For this review, use the dimensioned drawing (mm, ordinates from the lowest corner) and the shaded views. A direction names the side the tool comes from. Coordinates: 2 decimals unless noted, no trailing zeros. Loops run counter-clockwise (first coordinate to the right, second up) from the corner with the lowest first, then second, coordinate; pieces in that order, holes last. Notation, with made-up numbers: M 37,22 L 69,22 A24 ccw 69,38 Z; hole C -25,47 d10. An arc over 180 degrees is marked long. Write item = value, one per line.
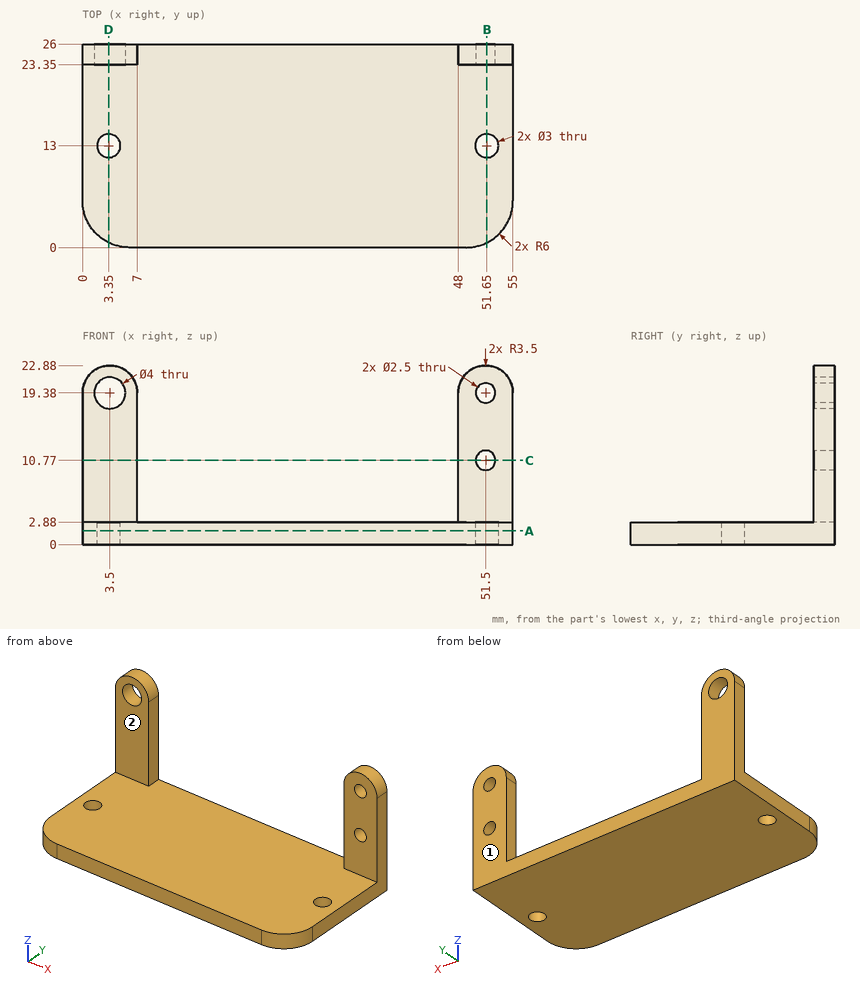
Q1. Machinability: for the marked faces 1 and 2, which of the approach directions +Z, -Z, +X, -X, +Y, -Y give a long, thin tool a straight path to every point of the face, cutting with its end or side? Answer none if there is none.
Solved:
face_1 = +Z, -Z, +X, -X, +Y
face_2 = +Z, +X, -X, -Y
Q2. Add section A-A (z = 1.75). Write out the cut boundary in (x, y), and give its area (3 significant figures).
Solved:
outline = M 0,6 A6 ccw 6,0 L 49,0 A6 ccw 55,6 L 55,26 L 0,26 Z; hole C 3.35,13 d3; hole C 51.65,13 d3
area = 1,400 mm²
Q3. For line 1 along Z through (x, y) = (51.5, 24.85); line 2 along Z through (x, y) = (45, 16); line 3 along Z through (x, y) = (3.5, 24.65), list the stretches that pass through material, from the lowest coordinate up.
Solved:
line_1 = 0 to 9.52, 12.02 to 18.13, 20.63 to 22.88
line_2 = 0 to 2.88
line_3 = 0 to 17.38, 21.38 to 22.88
Q4. For pin 1 Ø5 at (x, y) = (16, 12.5) entering from +Z; pin 2 Ø2 at (x, z) = (51.5, 16) entering from -Y; pin 3 Ø10 at (y, z) = (16, 15) entering from +X, all flat-tipped, find the tip position at first contact; note any pin that passes through.
Solved:
pin_1 = 2.88
pin_2 = 23.35
pin_3 = through
Q5. Add section C-C (z = 10.77). Write out the cut boundary in (x, y), and give its area (3 significant figures).
Solved:
outline = M 0,23.35 L 7,23.35 L 7,26 L 0,26 Z; M 48,23.35 L 50.25,23.35 L 50.25,26 L 48,26 Z; M 52.75,23.35 L 55,23.35 L 55,26 L 52.75,26 Z
area = 30.5 mm²
Q6. Add section D-D (x = 3.35). Write out the cut boundary in (y, z), and give its area (3 significant figures).
Solved:
outline = M 0.62,0 L 11.5,0 L 11.5,2.88 L 0.62,2.88 Z; M 14.5,0 L 26,0 L 26,17.39 L 23.35,17.39 L 23.35,2.88 L 14.5,2.88 Z; M 23.35,21.37 L 26,21.37 L 26,22.88 L 23.35,22.88 Z
area = 107 mm²
Q7. Add section B-B (x = 51.65). Write out the cut boundary in (y, z).
Solved:
outline = M 0.62,0 L 11.5,0 L 11.5,2.88 L 0.62,2.88 Z; M 14.5,0 L 26,0 L 26,9.53 L 23.35,9.53 L 23.35,2.88 L 14.5,2.88 Z; M 23.35,12.01 L 26,12.01 L 26,18.14 L 23.35,18.14 Z; M 23.35,20.62 L 26,20.62 L 26,22.88 L 23.35,22.88 Z
